The model under review builds one solid part; all positions refer to its coordinate system, in mm. Face numbers are marked on the shaded views. A direction names the side the tool comes from. Coordinates: 2 decimals unless noted, no trailing zeros. Write each loop counter-clockwise with the first axis right and the second up, starting at its lowest first coordinate (ties: lowest second). Pieces come first, ordered by that corner, then holes.
Autodesk Inventor part; units mm, degrees
ref_plane "YZ Plane" through (0, 0, 0) normal (1, 0, 0) x (0, 1, 0)
ref_plane "XZ Plane" through (0, 0, 0) normal (0, 1, 0) x (-1, 0, 0)
ref_plane "XY Plane" through (0, 0, 0) normal (0, 0, 1) x (1, 0, 0)
sketch "Sketch4" plane through (0, 0, 0) normal (0, 1, 0) x (-1, 0, 0)
  line L0 (-6.35, -28.956) -> (6.35, -28.956)
  line L1 (6.35, -28.956) -> (6.35, 28.956)
  line L2 (6.35, 28.956) -> (-6.35, 28.956)
  line L3 (-6.35, 28.956) -> (-6.35, -28.956)
  line L4 (-6.35, -28.956) -> (6.35, 28.956) construction
  line L5 (6.35, -28.956) -> (-6.35, 28.956) construction
  point P0 (0, 0)
  dimension "d14" = 12.7
  dimension "d15" = 57.912
extrude "Extrusion3" add sketch "Sketch4" along normal blind 7.62
sketch "Sketch5" plane through (-6.35, 0, -28.956) normal (-1, 0, 0) x (0, 0, 1)
  line L0 (0, 0) -> (57.912, 0)
  line L1 (57.912, 0) -> (57.912, 7.62)
  line L2 (0, 7.62) -> (57.912, 7.62)
  line L3 (0, 7.62) -> (7.62, 7.62)
  line L4 (7.62, 7.62) -> (7.62, 0)
  line L5 (7.62, 0) -> (0, 0)
  line L6 (0, 0) -> (0, 7.62)
  line L7 (57.15, 0) -> (50.8, 0)
  line L8 (50.8, 0) -> (50.8, 7.62)
  line L9 (50.8, 7.62) -> (57.912, 7.62)
  line L10 (57.912, 0) -> (57.15, 0)
  point P0 (28.956, 0)
  dimension "d18" = 7.62
  dimension "d21" = 50.8
extrude "Extrusion4" add sketch "Sketch5" along normal blind 20.32 contours L6 L2 L4 L0 | L8 L2 L1 L0
sketch "Sketch6" plane through (0, 7.62, 0) normal (0, 1, 0) x (1, 0, 0)
  line L0 (6.35, -28.956) -> (-26.67, -28.956)
  line L1 (6.35, -28.956) -> (6.35, 28.956)
  line L2 (-22.7838, 26.9211) -> (-22.7838, -27.5281) construction
  line L3 (-10.1854, 26.9211) -> (-10.1854, -27.5281) construction
  line L4 (-7.0821, 25.146) -> (-30.0582, 25.146) construction
  line L5 (-5.6948, -25.4) -> (-30.0582, -25.4) construction
  point P0 (-26.67, 28.956)
  point P1 (-26.67, 21.336)
  point P2 (-26.67, -21.844)
  point P3 (0, 0)
  point P4 (-22.7838, 25.146)
  point P5 (-10.1854, 25.146)
  point P6 (-10.1854, -25.4)
  point P7 (-22.7838, -25.4)
  dimension "d26" = 3.556
  dimension "d27" = 3.81
  dimension "d28" = 3.8862
  dimension "d29" = 12.5984
  dimension "d30" = 16.4846
hole "Hole1" at (-22.7838, 7.62, -25.146) at (-10.1854, 7.62, -25.146) at (-10.1854, 7.62, 25.4) at (-22.7838, 7.62, 25.4) direction (0, -1, 0) diameter 3.6576 end up to surface
sketch "Sketch7" plane through (6.35, 0, 28.956) normal (0, 0, 1) x (1, 0, 0)
  line L0 (0, 0) -> (-33.02, 0)
  line L1 (0, 0) -> (0, 7.62)
  line L2 (0, 7.62) -> (-33.02, 7.62)
  line L3 (-12.7, 0) -> (-12.7, 7.62)
  line L4 (-12.7, 7.62) -> (-12.7, 0)
  line L5 (-6.5931, 0) -> (-6.5931, 7.62) construction
  line L6 (-12.7, 3.81) -> (-6.5931, 3.81) construction
  line L7 (0, 3.81) -> (-6.5931, 3.81) construction
  point P0 (-6.35, 0)
  point P1 (-9.6465, 3.81)
  point P2 (-3.2965, 3.81)
  dimension "d38" = 6.5931
hole "Hole2" at (-3.2965, 3.81, 28.956) at (3.0535, 3.81, 28.956) direction (0, 0, -1) diameter 2.6416 depth 12.7 tip angle 118
properties part number "servo_mount" material "Aluminum 6061"
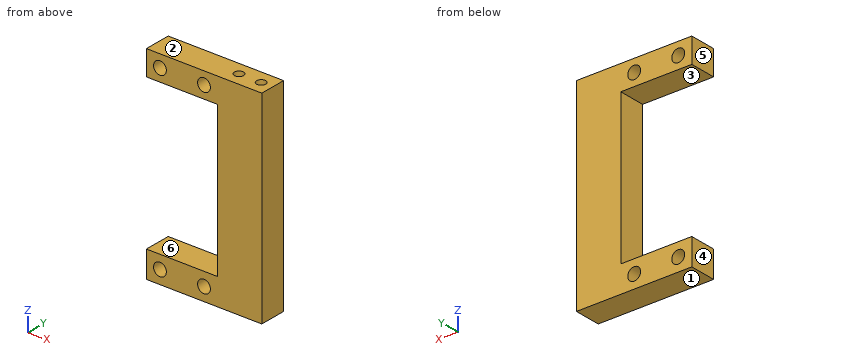
Item 1: To check wall thickness, follow line 1 along X through (y, z) = (5.5, 25.4) (3 decimals); line 2 along X through (y, z) = (3.81, 22.25); line 3 along Z through (x, y) = (-19.5, 3.75). State the ranges of each line that lie inside material, in increasing order.
Solved:
line 1: x = -26.67 to -24.613, -20.955 to -12.014, -8.357 to 6.35
line 2: x = -26.67 to -4.62, -1.98 to 1.73, 4.37 to 6.35
line 3: z = -28.96 to -21.34, 21.84 to 28.96
Item 2: Take a section at D-D, the plane x = -9. Write out the cut boundary in (y, z), plus the area to 3 significant figures.
Solved:
outline: (0, -28.96) - (7.62, -28.96) - (7.62, -26.54) - (0, -26.54) - close; (0, -23.75) - (7.62, -23.75) - (7.62, -21.34) - (0, -21.34) - close; (0, 21.84) - (7.62, 21.84) - (7.62, 24.01) - (0, 24.01) - close; (0, 26.79) - (7.62, 26.79) - (7.62, 28.96) - (0, 28.96) - close
area: 69.8 mm2
Item 3: Take a section at B-B, the plane z = 25.4. Count the separate pieces of the cut face and the enclosed holes in it, plus the area to 3 significant figures.
Solved:
separate pieces: 3
enclosed holes: 2
area: 185 mm2
Item 4: Take a section at A-A, the plane x = -13.5. Write out the cut boundary in (y, z).
Solved:
outline: (0, -28.96) - (7.62, -28.96) - (7.62, -21.34) - (0, -21.34) - close; (0, 21.84) - (7.62, 21.84) - (7.62, 28.96) - (0, 28.96) - close
Item 5: Take a section at C-C, the plane y = 6.25. Write out the cut boundary in (x, z), plus the area to 3 significant figures.
Solved:
outline: (-26.67, -28.96) - (6.35, -28.96) - (6.35, 28.96) - (-26.67, 28.96) - (-26.67, 21.84) - (-6.35, 21.84) - (-6.35, -21.34) - (-26.67, -21.34) - close; hole circle Ø3.66 at (-22.78, -25.15); hole circle Ø3.66 at (-22.78, 25.4); hole circle Ø3.66 at (-10.19, -25.15); hole circle Ø3.66 at (-10.19, 25.4)
area: 993 mm2
Item 6: Machinability: for the marked faces 5 and 6, which of the approach directions +Z, -Z, +X, -X, +Y, -Y give a long, thin tool a straight path to every point of the face, cutting with its end or side? Answer none if there is none.
Solved:
face 5: +Z, -Z, -X, +Y, -Y
face 6: -X, +Y, -Y
Item 7: Mouldability with a two-part tool opening along Z and no side actions: class the marked faces 1, 2, 3 and 4 as pulls with the +Z half, pulls with the -Z half, needs draft (parallel to the pull), parting line crosses it, or undercut.
Solved:
face 1: pulls with the -Z half
face 2: pulls with the +Z half
face 3: undercut
face 4: needs draft
Item 8: For pin 1 (4 mm diameter, centred on x = -10.19, z = -25.15, fed in from +Y); pin 2 (2.5 mm diameter, centred on y = 3.5, z = -4, fed in from -X), all flat-tipped, find the tip position at first contact; note any pin that passes through.
Solved:
pin 1: stops at y = 7.62
pin 2: stops at x = -6.35
